The figure shows three views and two pictorial views of one solid part (mm, origin at its lowest corner). Answer the questions. Give positions to 0.01 mm unless a question says otherwise; leave off trailing zeros. Loops run counter-clockwise (first coordinate to the right, second up) from the corner with the lowest first, then second, coordinate; pieces in that order, holes last. Notation, with made-up numbers: M 76.25,4 L 113.25,4 A12 ccw 113.25,23 Z; hole C 34,5.5 d4. An arc over 180 degrees is marked long. Answer in a Markdown table with one row per item. Add a question column.
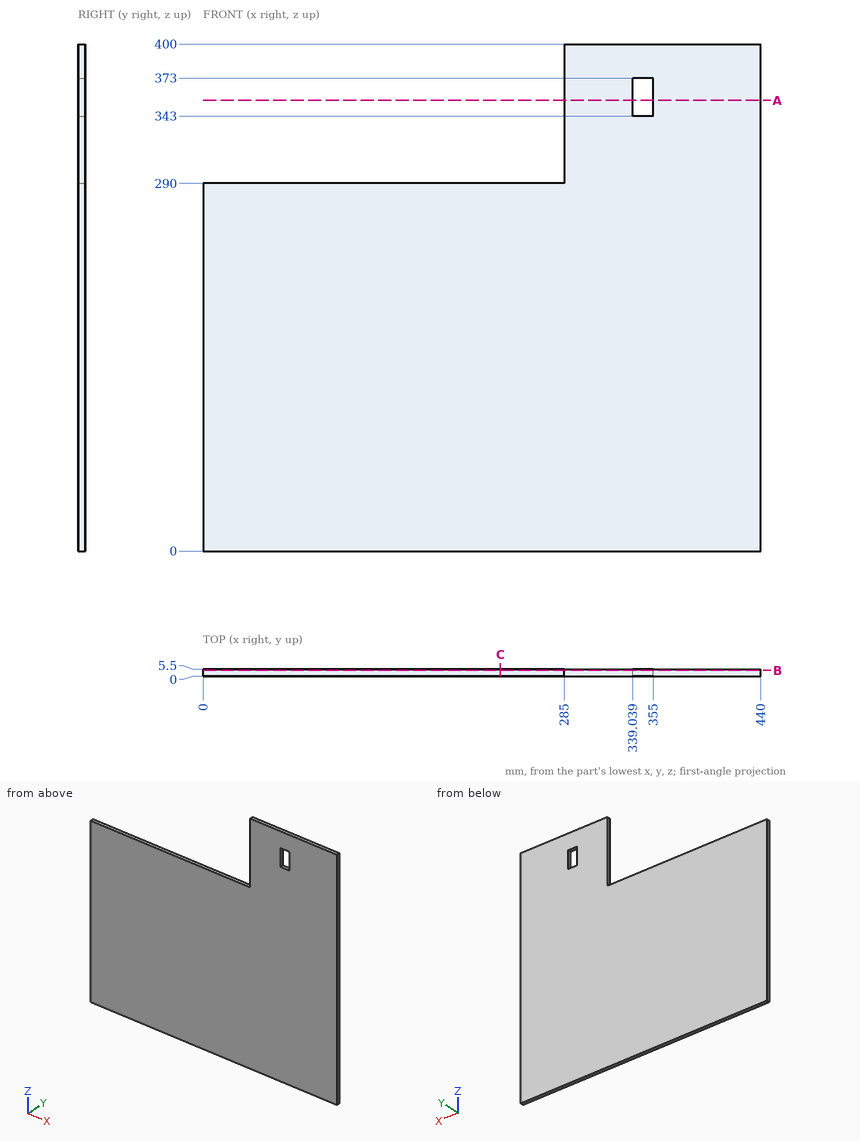
(1) Section A-A, the plane z = 355.5 is taken. Determine the outline of the cut face in (x, y).
(2) Section B-B, the plane y = 4.45 is taken. Determine the outline of the cut face in (x, z).
(3) Section C-C, the plane x = 234.5 is taken. Determine the outline of the cut face in (y, z).
(4) Each of these flat-tipped pins is pushed along its axis until it touches: P1, Ø1.6, axis at y = 4, z = 353.5, coming from the -X side; P2, Ø1, axis at x = 151, z = 228, coming from the -Y side; P3, Ø1.5, axis at x = 212.5, y = 3, coming from the +Z side. Where does it stop, or does it pass through?
(5) Consider line 1 along Z through (x, y) = (42.5, 3.55); line 2 along X through (y, z) = (0.9, 291.5). Determine where each line is inside the solid, lowest interval first. Write a range as from..to.
Numbers:
| question | item | result |
|---|---|---|
| 1 | outline | M 285,0 L 339.04,0 L 339.04,5.5 L 285,5.5 Z; M 355,0 L 440,0 L 440,5.5 L 355,5.5 Z |
| 2 | outline | M 0,0 L 440,0 L 440,400 L 285,400 L 285,290 L 0,290 Z; hole M 339.04,343 L 355,343 L 355,373 L 339.04,373 Z |
| 3 | outline | M 0,0 L 5.5,0 L 5.5,290 L 0,290 Z |
| 4 | P1 | stops at x = 285 |
| 4 | P2 | stops at y = 0 |
| 4 | P3 | stops at z = 290 |
| 5 | line 1 | z = 0..290 |
| 5 | line 2 | x = 285..440 |
